```python
from build123d import *

# Parameters (mm, degrees)
SKETCH_1_W      = 53
SKETCH_1_H      = 50
EXTRUDE_1_DEPTH = 3
SKETCH_2_W      = 51
SKETCH_2_H      = 50
SKETCH_2_R      = 11.05
SKETCH_2_R_2    = 1.6
EXTRUDE_2_DEPTH = 3
CHAMFER_1_SIZE  = 5


with BuildPart() as part:
    # 草图1 → 凸台-拉伸1 (new body)
    with BuildSketch(Plane.XY):
        with Locations((26.5, 25)):
            Rectangle(SKETCH_1_W, SKETCH_1_H)
        with BuildLine():
            Line((12, 42.1), (42, 42.1))
            ThreePointArc((42, 42.1), (44.1, 40), (42, 37.9))
            Line((42, 37.9), (12, 37.9))
            ThreePointArc((12, 37.9), (9.9, 40), (12, 42.1))
        make_face(mode=Mode.SUBTRACT)
        with BuildLine():
            Line((12, 7.9), (42, 7.9))
            ThreePointArc((42, 7.9), (44.1, 10), (42, 12.1))
            Line((42, 12.1), (12, 12.1))
            ThreePointArc((12, 12.1), (9.9, 10), (12, 7.9))
        make_face(mode=Mode.SUBTRACT)
    extrude(amount=EXTRUDE_1_DEPTH)

    # 草图2 → 凸台-拉伸2 (add)
    with BuildSketch(Plane.ZY):
        with Locations((25.5, 25)):
            Rectangle(SKETCH_2_W, SKETCH_2_H)
        with Locations((30, 25)):
            Circle(SKETCH_2_R, mode=Mode.SUBTRACT)
        with Locations((45.5, 40.5)):
            Circle(SKETCH_2_R_2, mode=Mode.SUBTRACT)
        with Locations((45.5, 9.5)):
            Circle(SKETCH_2_R_2, mode=Mode.SUBTRACT)
        with Locations((14.5, 9.5)):
            Circle(SKETCH_2_R_2, mode=Mode.SUBTRACT)
        with Locations((14.5, 40.5)):
            Circle(SKETCH_2_R_2, mode=Mode.SUBTRACT)
    extrude(amount=-EXTRUDE_2_DEPTH)

    # 倒角1
    chamfer_1_edges = [part.edges().sort_by_distance(p)[0] for p in [
        (1.5, 0, 51),
        (1.5, 50, 51),
        (53, 50, 1.5),
        (53, 0, 1.5),
    ]]
    chamfer(chamfer_1_edges, length=CHAMFER_1_SIZE)


solid = part.part
```
The model under review builds one solid part; all positions refer to its coordinate system, in mm. A direction names the side the tool comes from. Give positions to 0.01 mm unless a question says otherwise; leave off trailing zeros. Write each loop counter-clockwise with the first axis right and the second up, starting at its lowest first coordinate (ties: lowest second). Pieces come first, ordered by that corner, then holes. Notation, with made-up numbers: (36, 26.25) -> (42, 26.25) arc R20 ccw to (42, 34.25) -> close; hole circle Ø1 at (0, 43). An arc over 180 degrees is marked (long way). Put each result on its own line as item: value.
(1) We need section D-D, the plane z = 30. Give the boundary of the cut face in (x, y).
Results are:
outline: (0, 0) -> (3, 0) -> (3, 13.95) -> (0, 13.95) -> close; (0, 36.05) -> (3, 36.05) -> (3, 50) -> (0, 50) -> close
(2) The part is to be moulded in two halves that separate along Z. For faces 4 (the cylindrical face through (9.9, 10, 1.5)), 5 (the cylindrical face through (1.48, 7.94, 45.15)), 6 (the flat face through (1, 25, 51)), say which applies: pulls with the +Z half, pulls with the -Z half, needs draft (parallel to the pull), parting line crosses it, or undercut.
Results are:
face 4: needs draft
face 5: undercut
face 6: pulls with the +Z half
(3) To check wall thickness, follow probe 1 along Y at (x, z) = (0.75, 45.5); probe 2 along Y at (x, z) = (1, 30); probe 3 along Y at (x, z) = (1, 14). State the ranges of each line that lie inside material, in increasing order. Write a range as from..to.
Results are:
probe 1: 0..7.9, 11.1..38.9, 42.1..50
probe 2: 0..13.95, 36.05..50
probe 3: 0..7.98, 11.02..38.98, 42.02..50
(4) We need section A-A, the plane z = 14.5. Give the boundary of the cut face in (x, y).
Results are:
outline: (0, 0) -> (3, 0) -> (3, 7.9) -> (0, 7.9) -> close; (0, 11.1) -> (3, 11.1) -> (3, 38.9) -> (0, 38.9) -> close; (0, 42.1) -> (3, 42.1) -> (3, 50) -> (0, 50) -> close
(5) For pin 1 Ø6 at (y, z) = (44.5, 42) entering from -X; pin 2 Ø4 at (y, z) = (9.5, 14.5) entering from +X, all flat-tipped, find the tip position at first contact; note any pin that passes through.
Results are:
pin 1: x = 0
pin 2: x = 3
(6) We need section C-C, the plane y = 31. Give the boundary of the cut face in (x, z).
Results are:
outline: (0, 0) -> (53, 0) -> (53, 3) -> (3, 3) -> (3, 20.72) -> (0, 20.72) -> close; (0, 39.28) -> (3, 39.28) -> (3, 51) -> (0, 51) -> close
(7) We need section B-B, the plane x = 17. Give the boundary of the cut face in (y, z), and give its area (3 significant figures).
Results are:
outline: (0, 0) -> (7.9, 0) -> (7.9, 3) -> (0, 3) -> close; (12.1, 0) -> (37.9, 0) -> (37.9, 3) -> (12.1, 3) -> close; (42.1, 0) -> (50, 0) -> (50, 3) -> (42.1, 3) -> close
area: 125 mm²
(8) Tool access review of faces 1 (the cylindrical face through (9.9, 40, 1.5)), 2 (the flat face through (28, 25, 3)), 3 (the cylindrical face through (1.48, 39.53, 13.23)): name each direction out of +Z, -Z, +X, -X, +Y, -Y from which nothing blocks a thin tool from reaching the whole face with its end or side.
Results are:
face 1: +Z, -Z
face 2: +Z, +X, +Y, -Y
face 3: +X, -X
